from build123d import *

# Parameters (mm, degrees)
SKETCH2_W          = 20
SKETCH2_H          = 20
CUT_EXTRUDE1_DEPTH = 25


with BuildPart() as part:
    # Sketch1 → Revolve1 (revolve)
    with BuildSketch(Plane(origin=(0, 0, 0), x_dir=(0, 0, -1), z_dir=(1, 0, 0))):
        Polygon((-25, 3), (-24.385665, 2.385665), (-1.317445659, 2.385665), (0, 3), (0, 5.75), (-25, 5.75), align=None)
    revolve(axis=Axis((0, 0, 0), (0, 0, 1)))

    # Sketch2 → Cut-Extrude1 (cut)
    with BuildSketch(Plane.XY):
        Rectangle(SKETCH2_W, SKETCH2_H)
        Polygon((-5, 2.886751346), (-5, -2.886751346), (0, -5.773502692), (5, -2.886751346), (5, 2.886751346), (0, 5.773502692), align=None, mode=Mode.SUBTRACT)
    extrude(amount=CUT_EXTRUDE1_DEPTH, mode=Mode.SUBTRACT)


solid = part.part
Here's how the part is built. I have some questions about the finished solid (model axes, mm). Round coordinates to 2 decimals unless told otherwise and drop trailing zeros. Loops run counter-clockwise (first coordinate to the right, second up) from the corner with the lowest first, then second, coordinate; pieces in that order, holes last.
1. If we section it at C-C on x = 3.5: Write out the boundary of the cut face in (y, z).
Answer list:
outline: (-3.75, 0) - (3.75, 0) - (3.75, 25) - (-3.75, 25) - close
2. If I drill on line 1 along Y through (x, z) = (0, 23); line 2 along X through (y, z) = (0, 7.5); line 3 along X through (y, z) = (2, 3.5), over which ranges is the centre line in solid material (lowest first)?
Answer list:
line 1: y = -5.75 to -2.39, 2.39 to 5.75
line 2: x = -5 to -2.39, 2.39 to 5
line 3: x = -5 to -1.3, 1.3 to 5
3. We'd pull the mould along Y, two halves only. Please class faces 1 (the face through (-2.466, 4.35, 12.325)), 2 (the face through (2.33, -0.52, 12.69)), 3 (the face through (2.466, -4.35, 12.325)): +Y half, -Y half, draft (parallel to the pull), parting line (faces both ways), or undercut.
Answer list:
face 1: +Y half
face 2: undercut
face 3: -Y half
4. For P1, Ø5.5, axis at x = 0, y = 0, coming from the -Z side, with a flat end and sliding along its axis, tell me the tip position at first contact or that it passes through.
Answer list:
P1: stops at z = 0.54
5. If we section it at B-B on z = 7.25: Write out the boundary of the cut face in (x, y).
Answer list:
outline: (-5, -2.84) arc R5.75 ccw to (-4.96, -2.91) - (-0.04, -5.75) arc R5.75 ccw to (0.04, -5.75) - (4.96, -2.91) arc R5.75 ccw to (5, -2.84) - (5, 2.84) arc R5.75 ccw to (4.96, 2.91) - (0.04, 5.75) arc R5.75 ccw to (-0.04, 5.75) - (-4.96, 2.91) arc R5.75 ccw to (-5, 2.84) - close; hole circle Ø4.77 at (0, 0)
6. If we section it at A-A on y = 0: Write out the boundary of the cut face in (x, z), plus the area to 3 significant figures.
Answer list:
outline: (-5, 0) - (-3, 0) - (-2.39, 1.32) - (-2.39, 24.39) - (-3, 25) - (-5, 25) - close; (2.39, 1.32) - (3, 0) - (5, 0) - (5, 25) - (3, 25) - (2.39, 24.39) - close
area: 130 mm2
